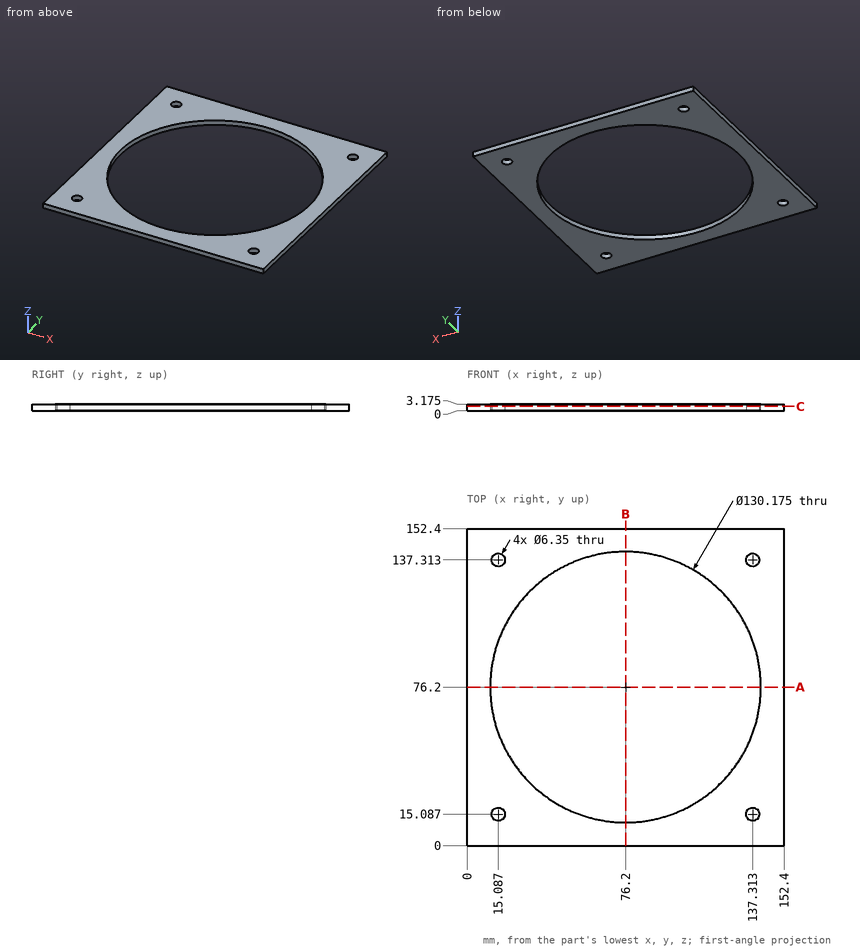
Check sheet for the drawn part. Datum: minimum x, y, z corner. Units: mm. Give positions to 0.01 mm unless a question says otherwise; leave off trailing zeros. Order: outer loops, then holes, each group sorted by start corner. A loop starts at its lowest first (then second) coordinate and runs counter-clockwise, first axis right, second up. Notation, with made-up numbers: (-36, -11) -> (0, -11) arc R11 ccw to (0, 8) -> close; hole circle Ø5 at (89, -16.75). An arc over 180 degrees is marked (long way). Return JSON: item names as keys, results as strings.
1. Material ranges on probe 1 along Y at (x, z) = (75, 2.75); probe 2 along Y at (x, z) = (34, 0.75); probe 3 along X at (y, z) = (19, 2), recorded low to high. Write a range as [from, to].
From the geometry:
{"probe 1": "[0, 11.12], [141.28, 152.4]", "probe 2": "[0, 26.65], [125.75, 152.4]", "probe 3": "[0, 45.14], [107.26, 152.4]"}
2. Cross-section at A-A, the plane y = 76.2. Record the cut outline in (x, z) (1 decimal).
From the geometry:
{"outline": "(0, 0) -> (11.1, 0) -> (11.1, 3.2) -> (0, 3.2) -> close; (141.3, 0) -> (152.4, 0) -> (152.4, 3.2) -> (141.3, 3.2) -> close"}
3. Go/stop test with a flat-tipped pin: P1, Ø5.5, axis at x = 137.31, y = 137.31, coming from the +Z side. Record where the tip stops, or that it passes through.
From the geometry:
{"P1": "through"}
4. Cross-section at C-C, the plane z = 2. Count the separate pieces of the cut face and the enclosed holes in it, plus the area to 3 significant figures.
From the geometry:
{"separate pieces": "1", "enclosed holes": "5", "area": "9,790 mm^2"}
